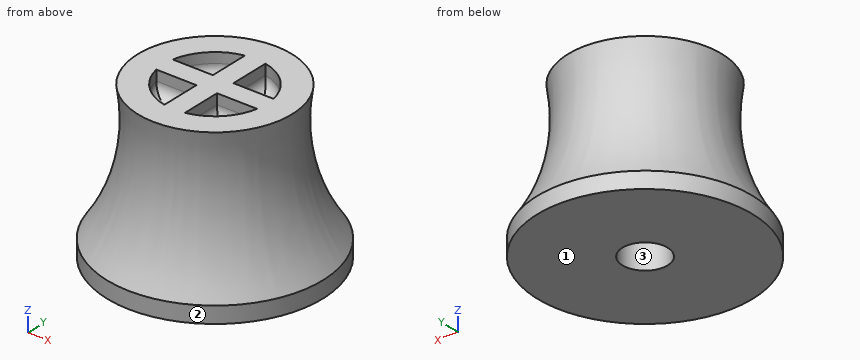
```python
from build123d import *

# Parameters (mm, degrees)
F2_R     = 1.1
F3_DEPTH = 5
F5_DEPTH = 1
F6_R     = 0.5


with BuildPart() as f1:
    # F0 (on Right) → F1 (revolve)
    with BuildSketch(Plane.YZ):
        with BuildLine():
            Line((-5.25, 0), (0, 0))
            Line((0, 0), (0, 7.5))
            Line((0, 7.5), (-3.75, 7.5))
            ThreePointArc((-3.75, 7.5), (-3.835993, 4.001342), (-5.25, 0.8))
            Line((-5.25, 0.8), (-5.25, 0))
        make_face()
    revolve(axis=Axis((0, 0, 7.262046), (0, 0, -1)))

    # F2 (on face) → F3 (cut)
    with BuildSketch(Plane(origin=(0, 0, 0), x_dir=(1, 0, 0), z_dir=(0, 0, -1))):
        Circle(F2_R)
    extrude(amount=-F3_DEPTH, mode=Mode.SUBTRACT)

    # F4 (on face) → F5 (cut)
    with BuildSketch(Plane.XY.offset(7.5)):
        with BuildLine():
            Line((-0.5, 0.5), (-0.5, 2.44949))
            ThreePointArc((-0.5, 2.44949), (-1.767767, 1.767767), (-2.44949, 0.5))
            Line((-2.44949, 0.5), (-0.5, 0.5))
        make_face()
        with BuildLine():
            ThreePointArc((2.44949, 0.5), (1.767767, 1.767767), (0.5, 2.44949))
            Line((0.5, 2.44949), (0.5, 0.5))
            Line((0.5, 0.5), (2.44949, 0.5))
        make_face()
        with BuildLine():
            Line((-0.5, -0.5), (-2.44949, -0.5))
            ThreePointArc((-2.44949, -0.5), (-1.767767, -1.767767), (-0.5, -2.44949))
            Line((-0.5, -2.44949), (-0.5, -0.5))
        make_face()
        with BuildLine():
            Line((0.5, -0.5), (0.5, -2.44949))
            ThreePointArc((0.5, -2.44949), (1.767767, -1.767767), (2.44949, -0.5))
            Line((2.44949, -0.5), (0.5, -0.5))
        make_face()
    extrude(amount=-F5_DEPTH, mode=Mode.SUBTRACT)

    # F6
    f6_edges = [f1.edges().sort_by_distance(p)[0] for p in [
        (-1.474745, 0.5, 6.5),
        (-0.5, 1.474745, 6.5),
        (-1.767767, 1.767767, 6.5),
        (1.767767, 1.767767, 6.5),
        (0.5, 1.474745, 6.5),
        (1.474745, 0.5, 6.5),
        (1.474745, -0.5, 6.5),
        (0.5, -1.474745, 6.5),
        (1.767767, -1.767767, 6.5),
        (-0.5, -1.474745, 6.5),
        (-1.474745, -0.5, 6.5),
        (-1.767767, -1.767767, 6.5),
    ]]
    fillet(f6_edges, radius=F6_R)


solid = f1.part
```
Input: part model. Units: mm. Frame: model coordinates. Face numbers are marked on the shaded views. Give positions to 0.01 mm unless a question says otherwise; leave off trailing zeros. Write each loop counter-clockwise with the first axis right and the second up, starting at its lowest first coordinate (ties: lowest second). Pieces come first, ordered by that corner, then holes. Notation, with made-up numbers: (-20.5, -19.75) - (15.5, -19.75) arc R13 cw to (15.5, -1.75) - close; hole circle Ø8 at (-21.5, 75). An arc over 180 degrees is marked (long way). Write item = value, one per line. Start each with the question number.
1) Pin query (flat end, axial travel): pin 1 (2.5 mm diameter, centred on x = 0, y = 0.5, fed in from -Z); pin 2 (0.6 mm diameter, centred on y = -1.5, z = 7, fed in from +X); pin 3 (0.6 mm diameter, centred on x = -1, z = 7, fed in from +Y); pin 4 (0.6 mm diameter, centred on y = -2, z = 7, fed in from -X). Return the tip coordinate at first contact, or that it passes through.
2) Cut plane B-B (z = 6.75). Return loops of the section in (x, y), and give its area (3 significant figures).
3) Cut plane D-D (z = 2). Return loops of the section in (x, y).
4) Material intervals for L1, parallel to X at y = -1.5, z = 7.25; L2, parallel to X at y = 0, z = 2.45; L3, parallel to X at y = -0.5, z = 0.75, sorted ascending. Write a range as [from, to].
5) Draft query along X for the marked faces 1, 2 and 3. Return one class per face: pulls with the +X half, pulls with the -X half, needs draft (parallel to the pull), parting line crosses it, or undercut.
6) Cut plane A-A (x = 0). Return loops of the section in (y, z).
Answers follow:
q1.pin_1 = 0
q1.pin_2 = 3.48
q1.pin_3 = 3.62
q1.pin_4 = -3.27
q2.outline = circle Ø7.31 at (0, 0); hole (-2.37, -0.57) arc R2.43 ccw to (-0.57, -2.37) - (-0.57, -0.57) - close; hole (-2.37, 0.57) - (-0.57, 0.57) - (-0.57, 2.37) arc R2.43 ccw to start; hole (0.57, -2.37) arc R2.43 ccw to (2.37, -0.57) - (0.57, -0.57) - close; hole (0.57, 0.57) - (2.37, 0.57) arc R2.43 ccw to (0.57, 2.37) - close
q2.area = 33.0 mm^2
q3.outline = circle Ø9.08 at (0, 0); hole circle Ø2.2 at (0, 0)
q4.L1 = [-3.39, -2], [-0.5, 0.5], [2, 3.39]
q4.L2 = [-4.33, -1.1], [1.1, 4.33]
q4.L3 = [-5.23, -0.98], [0.98, 5.23]
q5.face_1 = needs draft
q5.face_2 = parting line crosses it
q5.face_3 = undercut
q6.outline = (-5.25, 0) - (-1.1, 0) - (-1.1, 5) - (1.1, 5) - (1.1, 0) - (5.25, 0) - (5.25, 0.8) arc R9 cw to (3.75, 7.5) - (-3.75, 7.5) arc R9 cw to (-5.25, 0.8) - close
